Model file for the job. Use its own axes, mm. Face numbers are marked on the shaded views. A direction names the side the tool comes from. Round coordinates to 2 decimals unless told otherwise and drop trailing zeros. Loops run counter-clockwise (first coordinate to the right, second up) from the corner with the lowest first, then second, coordinate; pieces in that order, holes last. Notation, with made-up numbers: (17.5, 56) -> (45.5, 56) arc R22 cw to (45.5, 81) -> close; hole circle Ø7 at (36.25, 32). An arc over 180 degrees is marked (long way). Use a Markdown table: item, result.
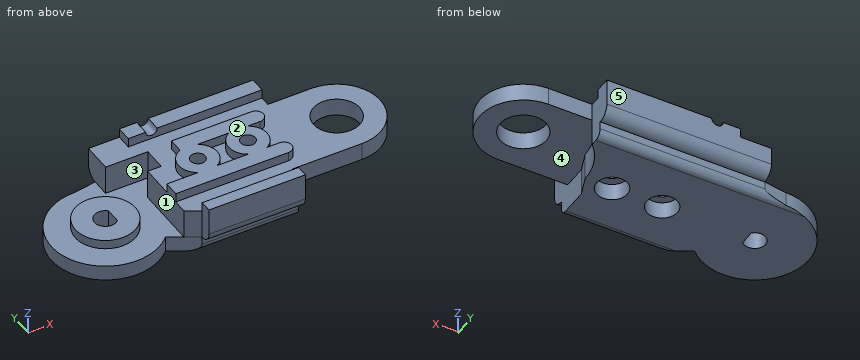
from build123d import *

# Parameters (mm, degrees)
BOSS_EXTRUDE1_DEPTH = 2
BOSS_EXTRUDE2_DEPTH = 1.5
BOSS_EXTRUDE3_DEPTH = 2.3
SKETCH6_W           = 5.48
SKETCH6_H           = 3
CUT_EXTRUDE1_DEPTH  = 3.8
SKETCH7_R           = 3
CUT_EXTRUDE2_DEPTH  = 3.3
SKETCH8_W           = 17.343145751
SKETCH8_H           = 2
SKETCH8_W_2         = 12.500252532
SKETCH8_H_2         = 1.5
BOSS_EXTRUDE4_DEPTH = 1.2
SKETCH9_R           = 2.5
BOSS_EXTRUDE5_DEPTH = 1.2
SKETCH10_R          = 0.95
CUT_EXTRUDE3_DEPTH  = 8.2
SKETCH11_R          = 2
CUT_EXTRUDE4_DEPTH  = 2.2
SKETCH12_R          = 3.9
BOSS_EXTRUDE6_DEPTH = 1.2
CUT_EXTRUDE5_DEPTH  = 3.2
FILLET1_R           = 1.5
FILLET2_R           = 1
SKETCH15_R          = 0.75
CUT_EXTRUDE6_DEPTH  = 4


with BuildPart() as part:
    # Sketch2 → Boss-Extrude1 (new body)
    with BuildSketch(Plane.XY):
        with BuildLine():
            Line((0, 7), (3, 7.456854249))
            Line((3, 7.456854249), (24.343145751, 7.456854249))
            Line((24.343145751, 7.456854249), (24.343145751, 5.656854249))
            ThreePointArc((24.343145751, 5.656854249), (22.60896374, 3.061467459), (22, 0))
            Line((22, 0), (21, -2.543145751))
            Line((21, -2.543145751), (21, -7.043145751))
            Line((21, -7.043145751), (8.499747468, -7.043145751))
            Line((8.499747468, -7.043145751), (4.949747468, -4.949747468))
            ThreePointArc((4.949747468, -4.949747468), (-6.467156728, -2.678784027), (0, 7))
        make_face()
    extrude(amount=BOSS_EXTRUDE1_DEPTH)

    # Sketch3 → Boss-Extrude2 (add)
    with BuildSketch(Plane.XY.offset(2)):
        with BuildLine():
            Line((24.343145751, 7.456854249), (24.343145751, 5.656854249))
            ThreePointArc((24.343145751, 5.656854249), (22.60896374, 3.061467459), (22, 0))
            Line((22, 0), (21, -2.543145751))
            Line((21, -2.543145751), (21, -7.043145751))
            Line((21, -7.043145751), (21, -8.543145751))
            Line((21, -8.543145751), (8.499747468, -8.543145751))
            Line((8.499747468, -8.543145751), (8.499747468, -7.043145751))
            Line((8.499747468, -7.043145751), (6.724747468, -5.996446609))
            Line((6.724747468, -5.996446609), (6.724747468, 2.126854249))
            Line((6.724747468, 2.126854249), (3, 2.126854249))
            Line((3, 2.126854249), (3, 7.456854249))
            Line((3, 7.456854249), (3, 8.956854249))
            Line((3, 8.956854249), (24.343145751, 8.956854249))
            Line((24.343145751, 8.956854249), (24.343145751, 7.456854249))
        make_face()
    extrude(amount=BOSS_EXTRUDE2_DEPTH)

    # Sketch5 → Boss-Extrude3 (add)
    with BuildSketch(Plane.XY.offset(3.5)):
        with BuildLine():
            Line((3, 7.5), (3, 2.126854249))
            Line((3, 2.126854249), (6.724747468, 2.126854249))
            Line((6.724747468, 2.126854249), (6.724747468, -5.996446609))
            Line((6.724747468, -5.996446609), (8.499747468, -7.043145751))
            Line((8.499747468, -7.043145751), (8.499747468, -8.543145751))
            Line((8.499747468, -8.543145751), (21, -8.543145751))
            Line((21, -8.543145751), (21, -5.656854249))
            Line((21, -5.656854249), (30.003145751, -5.656854249))
            ThreePointArc((30.003145751, -5.656854249), (35.66, 0), (30.003145751, 5.656854249))
            Line((30.003145751, 5.656854249), (24.343145751, 5.656854249))
            Line((24.343145751, 5.656854249), (24.343145751, 7.5))
            Line((24.343145751, 7.5), (24.343145751, 8.956854249))
            Line((24.343145751, 8.956854249), (3, 8.956854249))
            Line((3, 8.956854249), (3, 7.5))
        make_face()
    extrude(amount=BOSS_EXTRUDE3_DEPTH)

    # Sketch6 → Cut-Extrude1 (cut)
    with BuildSketch(Plane.XY.offset(5.8)):
        with Locations((5.74, 3.626854249)):
            Rectangle(SKETCH6_W, SKETCH6_H)
    extrude(amount=-CUT_EXTRUDE1_DEPTH, mode=Mode.SUBTRACT)

    # Sketch7 → Cut-Extrude2 (cut)
    with BuildSketch(Plane.XY.offset(5.8)):
        with Locations((30.003145751, 0)):
            Circle(SKETCH7_R)
    extrude(amount=-CUT_EXTRUDE2_DEPTH, mode=Mode.SUBTRACT)

    # Sketch8 → Boss-Extrude4 (add)
    with BuildSketch(Plane.XY.offset(5.8)):
        with Locations((15.671572876, 7.956854249)):
            Rectangle(SKETCH8_W, SKETCH8_H)
        with Locations((14.749873734, -7.793145751)):
            Rectangle(SKETCH8_W_2, SKETCH8_H_2)
        with BuildLine():
            Line((6.724747468, -4.172114809), (21.343145751, -4.172114809))
            ThreePointArc((21.343145751, -4.172114809), (22.343145751, -3.172114809), (21.343145751, -2.172114809))
            Line((21.343145751, -2.172114809), (6.724747468, -2.172114809))
            Line((6.724747468, -2.172114809), (6.724747468, -4.172114809))
        make_face()
        with BuildLine():
            Line((21.343145751, 4.180295218), (11, 4.180295218))
            Line((11, 4.180295218), (11, 2.180295218))
            Line((11, 2.180295218), (21.343145751, 2.180295218))
            ThreePointArc((21.343145751, 2.180295218), (22.343145751, 3.180295218), (21.343145751, 4.180295218))
        make_face()
    extrude(amount=BOSS_EXTRUDE4_DEPTH)

    # Sketch9 → Boss-Extrude5 (add)
    with BuildSketch(Plane.XY.offset(5.8)):
        with Locations((18.5, 0)):
            Circle(SKETCH9_R)
        with Locations((12, 0)):
            Circle(SKETCH9_R)
    extrude(amount=BOSS_EXTRUDE5_DEPTH)

    # Sketch10 → Cut-Extrude3 (cut)
    with BuildSketch(Plane.XY.offset(7)):
        with Locations((18.5, 0)):
            Circle(SKETCH10_R)
        with Locations((12, 0)):
            Circle(SKETCH10_R)
    extrude(amount=-CUT_EXTRUDE3_DEPTH, mode=Mode.SUBTRACT)

    # Sketch11 → Cut-Extrude4 (cut)
    with BuildSketch(Plane(origin=(0, 0, 0), x_dir=(-1, 0, 0), z_dir=(0, 0, -1))):
        with Locations((-12, 0)):
            Circle(SKETCH11_R)
        with Locations((-18.5, 0)):
            Circle(SKETCH11_R)
    extrude(amount=-CUT_EXTRUDE4_DEPTH, mode=Mode.SUBTRACT)

    # Sketch12 → Boss-Extrude6 (add)
    with BuildSketch(Plane.XY.offset(2)):
        Circle(SKETCH12_R)
    extrude(amount=BOSS_EXTRUDE6_DEPTH)

    # Sketch14 → Cut-Extrude5 (cut)
    with BuildSketch(Plane.XY.offset(3.2)):
        with BuildLine():
            Line((1, 0.979795897), (1, -0.979795897))
            ThreePointArc((1, -0.979795897), (-1.4, 0), (1, 0.979795897))
        make_face()
    extrude(amount=-CUT_EXTRUDE5_DEPTH, mode=Mode.SUBTRACT)

    # Fillet1
    fillet1_edges = [part.edges().sort_by_distance(p)[0] for p in [
        (13.671572875, 8.956854249, 2),
        (14.749873734, -8.543145751, 2),
    ]]
    fillet(fillet1_edges, radius=FILLET1_R - 0.0001)  # a hair under: the kernel refuses the full size

    # Fillet2
    fillet2_edges = [part.edges().sort_by_distance(p)[0] for p in [
        (14.749873734, -7.043145751, 0),
        (13.671572875, 7.456854249, 0),
    ]]
    fillet(fillet2_edges, radius=FILLET2_R)

    # Sketch15 → Cut-Extrude6 (cut)
    with BuildSketch(Plane.XZ.offset(-6.956854249)):
        with Locations((10, 7)):
            Circle(SKETCH15_R)
    extrude(amount=-CUT_EXTRUDE6_DEPTH, mode=Mode.SUBTRACT)


solid = part.part
Q1. Pull direction Y, two halves, no side cores. Call the marked faces 3, 4 and 5: released by +Y, released by -Y, zero draft, split by the parting line, or undercut.
Results list:
| item | result |
|---|---|
| face 3 | undercut |
| face 4 | zero draft |
| face 5 | released by +Y |
Q2. Flat gauge pins, fed straight in: pin 1 (3 mm diameter, centred on y = 2.5, z = 6, fed in from +X); pin 2 (2.5 mm diameter, centred on y = 3, z = 3.5, fed in from -X); pin 3 (1.1 mm diameter, centred on x = 5, z = 4.5, fed in from -Y). Where does each tip first touch, or does it go through?
Results list:
| item | result |
|---|---|
| pin 1 | stops at x = 35.57 |
| pin 2 | stops at x = -3.47 |
| pin 3 | stops at y = 5.13 |
Q3. Tool access for the marked faces 1 and 2: list every direction of +Z, -Z, +X, -X, +Y, -Y with a clear straight run to the whole face (end or side of a thin tool).
Results list:
| item | result |
|---|---|
| face 1 | +Z, -Y |
| face 2 | +Z, +X, -X, +Y, -Y |
Q4. Band-saw the part on A-A, the plane z = 5.25. Give the cut face in (x, y).
Results list:
| item | result |
|---|---|
| outline | (3, 5.13) -> (8.48, 5.13) -> (8.48, 2.13) -> (6.72, 2.13) -> (6.72, -6) -> (8.5, -7.04) -> (8.5, -8.54) -> (21, -8.54) -> (21, -5.66) -> (30, -5.66) arc R5.66 ccw to (30, 5.66) -> (24.34, 5.66) -> (24.34, 8.96) -> (3, 8.96) -> close; hole circle Ø1.9 at (12, 0); hole circle Ø1.9 at (18.5, 0); hole circle Ø6 at (30, 0) |
Q5. Drill centre lines: L1, parallel to Y at x = 12, z = 6.5; L2, parallel to Y at x = 0, z = 1.15; L3, parallel to Y at x = 12, z = 1.65. Where is each one in solid material? Low to high. Write a range as from..to.
Results list:
| item | result |
|---|---|
| L1 | y = -8.54..-7.04, -4.17..-0.95, 0.95..4.18, 6.96..8.96 |
| L2 | y = -7..-1.4, 1.4..7 |
| L3 | y = -7.04..-2, 2..7.46 |
